```python
from build123d import *

# Parameters (mm, degrees)
SKETCH1_W           = 50.8
SKETCH1_H           = 114.3
SKETCH1_R           = 1.27
BOSS_EXTRUDE1_DEPTH = 6.35
BOSS_EXTRUDE2_DEPTH = 50.8
SKETCH2_R           = 1.5
CUT_EXTRUDE1_DEPTH  = 12.7
FILLET1_R           = 2.54


with BuildPart() as part:
    # Sketch1 → Boss-Extrude1 (new, symmetric)
    with BuildSketch(Plane.XY):
        Rectangle(SKETCH1_W, SKETCH1_H)
        with Locations((0, 44.45)):
            Circle(SKETCH1_R, mode=Mode.SUBTRACT)
    extrude(amount=BOSS_EXTRUDE1_DEPTH, both=True)

    # Sketch3 → Boss-Extrude2 (add, through all)
    with BuildSketch(Plane(origin=(25.4, 0, 0), x_dir=(0, 0, -1), z_dir=(1, 0, 0))):
        Polygon((6.35, -57.15), (31.75, -57.15), (6.35, 19.05), align=None)
    extrude(amount=-BOSS_EXTRUDE2_DEPTH)

    # Sketch2 → Cut-Extrude1 (cut)
    with BuildSketch(Plane.XZ.offset(57.15)):
        with Locations(Location((-15.24, 0, 0), (0, 0, 270))):
            Circle(SKETCH2_R)
        with Locations(Location((15.24, 0, 0), (0, 0, 270))):
            Circle(SKETCH2_R)
        with Locations(Location((-15.24, -22.86, 0), (0, 0, 270))):
            Circle(SKETCH2_R)
        with Locations(Location((15.24, -22.86, 0), (0, 0, 270))):
            Circle(SKETCH2_R)
    extrude(amount=-CUT_EXTRUDE1_DEPTH, mode=Mode.SUBTRACT)

    # Fillet1
    fillet1_edges = [part.edges().sort_by_distance(p)[0] for p in [
        (-25.4, 0, 6.35),
        (25.4, 38.1, -6.35),
        (-25.4, -19.05, -19.05),
        (0, 19.05, -6.35),
        (25.4, -19.05, -19.05),
        (25.4, 0, 6.35),
        (-25.4, 38.1, -6.35),
        (0, 57.15, -6.35),
        (-25.4, 57.15, 0),
        (25.4, 57.15, 0),
        (0, 57.15, 6.35),
    ]]
    fillet(fillet1_edges, radius=FILLET1_R)


solid = part.part
```
For this review, take the finished solid that the model builds, in its own axes (mm). A direction names the side the tool comes from. Round coordinates to 2 decimals unless told otherwise and drop trailing zeros. Write each loop counter-clockwise with the first axis right and the second up, starting at its lowest first coordinate (ties: lowest second). Pieces come first, ordered by that corner, then holes. Notation, with made-up numbers: M 76.25,-37 L 123.25,-37 A32 cw 123.25,-4 Z; hole C 10,53.25 d1. An arc over 180 degrees is marked long. One line per item, written item: value. Start each with the question number.
(1) The part is to be moulded in two halves that separate along X. For faces 1 (the cylindrical face through (-24.636, -18.944, -18.251)), 2 (the cylindrical face through (0.32, 56.386, -5.626)), 3 (the flat face through (15, -44.45, 0)), say which applies: released by +X, released by -X, zero draft, split by the parting line, or undercut.
(2) We need section B-B (x = -7). Give the boundary of the cut face in (y, z).
(3) We need section A-A (y = 44.45). Give the boundary of the cut face in (x, z).
(4) We need section C-C (x = -15.24). Give the boundary of the cut face in (y, z).
(5) Insertion check: pin 1 (1.5 mm diameter, centred on x = -15, z = -23.5, fed in from -Y); pin 2 (2.5 mm diameter, centred on x = 15, z = -22, fed in from -Y). Each pin has a flat end and moves straight along its axis. Give the tip position at first contact, or say it passes through.
(6) Wall thickness on line 1 (X direction, y = -52.75, z = -22.86); line 2 (Y direction, x = 0, z = -1); line 3 (X direction, y = -53, z = -22): over which ranges is each line inside the solid? List them lowest first.
(7) Machinability: for faces 4 (the cylindrical face through (16.727, -50.889, 0.195)), 5 (the cylindrical face through (24.676, 37.282, -5.586)), 6 (the flat face through (0, 37, -6.35)), which of the approach directions +Z, -Z, +X, -X, +Y, -Y give a long, thin tool a straight path to every point of the face, cutting with its end or side? Answer none if there is none.
Result:
1. face 1: released by -X
1. face 2: zero draft
1. face 3: undercut
2. outline: M -57.15,-31.75 L 18.66,-6.48 A2.54 cw 19.46,-6.35 L 54.61,-6.35 A2.54 ccw 57.15,-3.81 L 57.15,3.81 A2.54 ccw 54.61,6.35 L -57.15,6.35 Z
3. outline: M -25.4,-3.81 A2.54 ccw -22.86,-6.35 L -1.27,-6.35 L -1.27,6.35 L -22.86,6.35 A2.54 ccw -25.4,3.81 Z; M 1.27,-6.35 L 22.86,-6.35 A2.54 ccw 25.4,-3.81 L 25.4,3.81 A2.54 ccw 22.86,6.35 L 1.27,6.35 Z
4. outline: M -57.15,-31.75 L 18.66,-6.48 A2.54 cw 19.46,-6.35 L 54.61,-6.35 A2.54 ccw 57.15,-3.81 L 57.15,3.81 A2.54 ccw 54.61,6.35 L -57.15,6.35 L -57.15,1.5 L -44.45,1.5 L -44.45,-1.5 L -57.15,-1.5 L -57.15,-21.36 L -44.45,-21.36 L -44.45,-24.36 L -57.15,-24.36 Z
5. pin 1: y = -44.45
5. pin 2: y = -57.15
6. line 1: -25.4 to -16.74, -13.74 to 13.74, 16.74 to 25.4
6. line 2: -57.15 to 43.18, 45.72 to 57.15
6. line 3: -25.4 to -16.47, -14.01 to 14.01, 16.47 to 25.4
7. face 4: -Y
7. face 5: -Z, +X, +Y
7. face 6: -Z, +X, -X, +Y
